Input: dimensioned drawing with shaded views. Units: mm. Origin: part minimum x, y, z. A direction names the side the tool comes from. Give positions to 0.01 mm unless a question says otherwise; leave off trailing zeros. Order: outer loops, then holes, each group sorted by start corner. A loop starts at its lowest first (then second) coordinate and runs counter-clockwise, first axis right, second up.
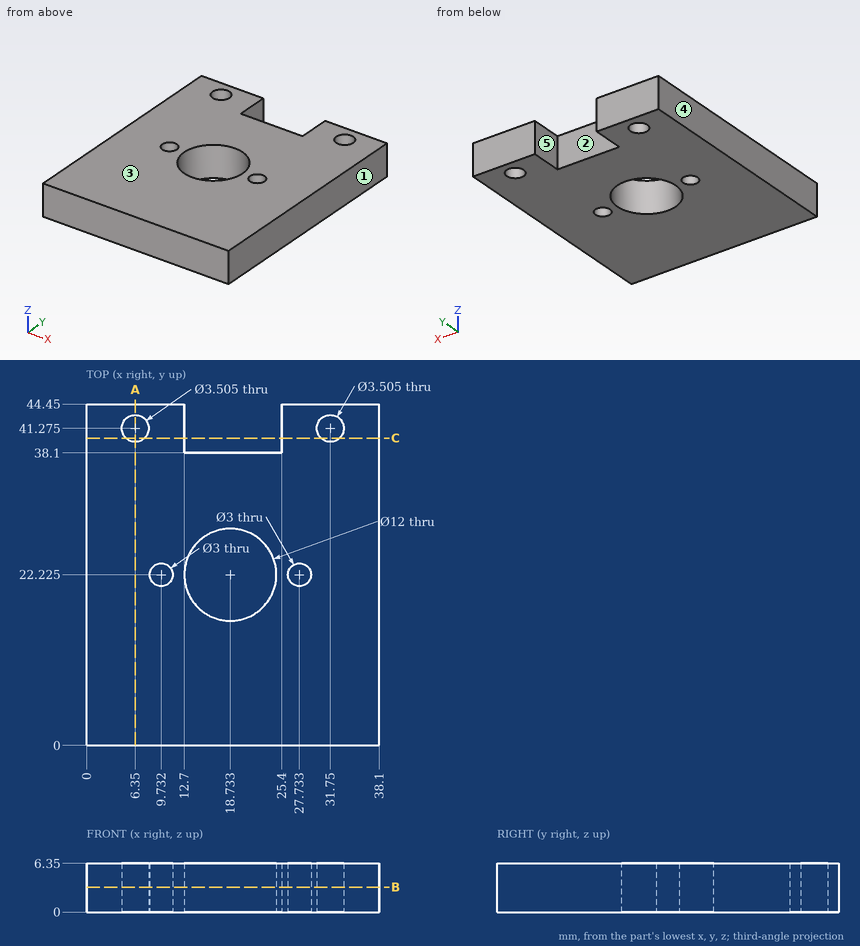
1) Material intervals for L1, parallel to Y at x = 6.35, z = 2.25; L2, parallel to X at y = 23.5, z = 1.75 (1 decimal); L3, parallel to Y at x = 16, z = 4 (1 decimal), sorted ascending.
Report:
L1: y = 0 to 39.52, 43.03 to 44.45
L2: x = 0 to 8.9, 10.5 to 12.9, 24.6 to 26.9, 28.5 to 38.1
L3: y = 0 to 16.9, 27.6 to 38.1
2) Section query A-A, the plane x = 6.35. Return the cut outline in (y, z), and give its area (3 significant figures).
Report:
outline: (0, 0) - (39.52, 0) - (39.52, 6.35) - (0, 6.35) - close; (43.03, 0) - (44.45, 0) - (44.45, 6.35) - (43.03, 6.35) - close
area: 260 mm2
3) Draft query along X for the marked faces 1, 2 and 3. Return one class per face: +X half, -X half, draft (parallel to the pull), parting line (faces both ways), or undercut.
Report:
face 1: +X half
face 2: undercut
face 3: draft
4) Reachability of the marked faces 4 and 5 from +Z, -Z, +X, -X, +Y, -Y: full face, straight path, thin tool, end or side. Return the list, or none.
Report:
face 4: +Z, -Z, -X, +Y, -Y
face 5: +Z, -Z, +Y
5) Section query B-B, the plane z = 3.25. Count the separate pieces of the cut face and the enclosed holes in it, and give its area (3 significant figures).
Report:
separate pieces: 1
enclosed holes: 5
area: 1,470 mm2
6) Section query C-C, the plane y = 40. Return the cut outline in (x, z), and give its area (3 significant figures).
Report:
outline: (0, 0) - (5.15, 0) - (5.15, 6.35) - (0, 6.35) - close; (7.55, 0) - (12.7, 0) - (12.7, 6.35) - (7.55, 6.35) - close; (25.4, 0) - (30.55, 0) - (30.55, 6.35) - (25.4, 6.35) - close; (32.95, 0) - (38.1, 0) - (38.1, 6.35) - (32.95, 6.35) - close
area: 131 mm2
7) Pin query (flat end, axial travel): pin 1 (1.8 mm diameter, centred on x = 9.73, y = 22.23, fed in from -Z); pin 2 (3 mm diameter, centred on x = 19.5, z = 4.5, fed in from +Y). Return the tip coordinate at first contact, or that it passes through.
Report:
pin 1: passes through
pin 2: stops at y = 38.1
